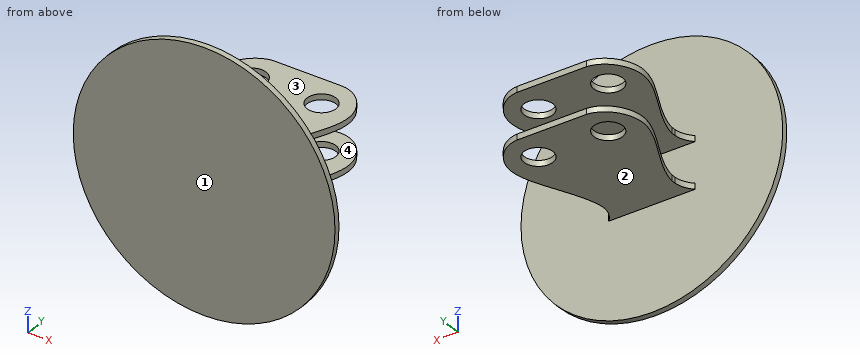
```python
from build123d import *

# Parameters (mm, degrees)
SKETCH1_R           = 45
BOSS_EXTRUDE1_DEPTH = 2
SKETCH2_W           = 12
SKETCH2_H           = 2
BOSS_EXTRUDE2_DEPTH = 50
BOSS_EXTRUDE3_START = -2
BOSS_EXTRUDE3_DEPTH = 2
SKETCH4_R           = 5
CUT_EXTRUDE1_DEPTH  = 50


# Read off the part's stored shape, not the designer's step: Boss-Extrude3
with BuildPart() as part:
    # Sketch1 → Boss-Extrude1 (new body)
    with BuildSketch(Plane(origin=(0, 0, 0), x_dir=(1, 0, 0), z_dir=(0, 1, 0))):
        with Locations(Location((0, 0, 0), (0, 0, 270))):
            Circle(SKETCH1_R)
    extrude(amount=BOSS_EXTRUDE1_DEPTH)

    # Sketch2 → Boss-Extrude2 (add)
    with BuildSketch(Plane(origin=(0, 2, 0), x_dir=(1, 0, 0), z_dir=(0, 1, 0))):
        with Locations((-6, -8)):
            Rectangle(SKETCH2_W, SKETCH2_H)
    extrude(amount=BOSS_EXTRUDE2_DEPTH)

    # Boss-Extrude3 outline → Boss-Extrude3 (add)
    with BuildSketch(Plane.XY.offset(9).offset(BOSS_EXTRUDE3_START)):
        with BuildLine():
            Line((-12, 9.252585755), (-12, 52))
            add(Edge.make_bspline(
                [(-12, 52), (-17.707608273, 51.500079533), (-24.252880777, 43.259732346), (-21.397540076, 31.962524142), (-17.33880503, 23.974508646), (-13.768744124, 16.530528707), (-12.117269051, 11.269699014), (-12, 9.252585755)],
                knots=[0, 0, 0, 0, 0.28798008, 0.430455664, 0.586456405, 0.756216635, 0.864299894, 0.864299894, 0.864299894, 0.864299894], degree=3))
        make_face()
        with BuildLine():
            Line((-12, 2), (-12, 7.979725632))
            add(Edge.make_bspline(
                [(-12, 7.979725632), (-12.129131204, 5.890942784), (-12.929877772, 3.858184366), (-14.891007751, 2)],
                knots=[0.887122224, 0.887122224, 0.887122224, 0.887122224, 1, 1, 1, 1], degree=3))
            Line((-14.891007751, 2), (-12, 2))
        make_face()
    extrude(amount=BOSS_EXTRUDE3_DEPTH)

    # Sketch4 → Cut-Extrude1 (cut)
    with BuildSketch(Plane.XY.offset(9)):
        with Locations((-12, 41.201646807)):
            Circle(SKETCH4_R)
    extrude(amount=-CUT_EXTRUDE1_DEPTH, mode=Mode.SUBTRACT)

    # Mirror1: part across plane


with BuildPart() as part_1:
    add(part.part)
    add(part.part.mirror(Plane(origin=(0, 52, 0), x_dir=(0, 0, 1), z_dir=(1, 0, 0))))

    # Mirror2: part across plane


with BuildPart() as part_2:
    add(part_1.part)
    add(part_1.part.mirror(Plane.XY))


solid = part_2.part
```
Geometry check sheet. Reference: the model listing, model coordinates, mm. Face numbers are marked on the shaded views. A direction names the side the tool comes from. Give positions to 0.01 mm unless a question says otherwise; leave off trailing zeros. Order: outer loops, then holes, each group sorted by start corner. A loop starts at its lowest first (then second) coordinate and runs counter-clockwise, first axis right, second up. Notation, with made-up numbers: (88.25, -31.75) - (147.25, -31.75) arc R24 ccw to (147.25, -19.75) - close; hole circle Ø8 at (5.25, -21.75). An arc over 180 degrees is marked (long way). Write item = value, one per line. Start each with the question number.
1) Section check A-A (x = 0). Enter the section's corners in (y, z).
2) Section check B-B (z = 0). Enter the section's corners in (x, y), then the cut area to 3 significant figures.
3) Section check C-C (x = -33). Enter the section's corners in (y, z).
4) Gauge pin test, flat ends, axial feed: pin 1 Ø1.5 at (x, y) = (-8, 24) entering from +Z; pin 2 Ø12 at (y, z) = (12.5, -6) entering from -X; pin 3 Ø4 at (x, y) = (1, 41) entering from -Z; pin 4 Ø6 at (x, y) = (-12, 41.2) entering from -Z. Record the tip position at first contact, or that the pin passes through.
5) Scan lines: L1, parallel to Z at x = 6, y = 47; L2, parallel to Y at x = 4.5, z = 3.5. Record each from-to range of solid material in increasing order.
6) Access from +Z, -Z, +X, -X, +Y, -Y to the whole of each face (thin tool, end or side, straight path). Record for the marked faces 1, 2, 3 and 4.
Geometry check:
q1.outline = (0, -45) - (2, -45) - (2, -9) - (52, -9) - (52, -7) - (2, -7) - (2, 7) - (52, 7) - (52, 9) - (2, 9) - (2, 45) - (0, 45) - close
q2.outline = (-45, 0) - (45, 0) - (45, 2) - (-45, 2) - close
q2.area = 180 mm2
q3.outline = (0, -30.59) - (2, -30.59) - (2, 30.59) - (0, 30.59) - close
q4.pin_1 = 9
q4.pin_2 = -14.77
q4.pin_3 = -9
q4.pin_4 = through
q5.L1 = -9 to -7, 7 to 9
q5.L2 = 0 to 2
q6.face_1 = +Z, -Z, +X, -X, -Y
q6.face_2 = -Z, +X, -X, +Y
q6.face_3 = +Z, +X, -X, +Y
q6.face_4 = +X, -X, +Y
